from build123d import *

# Parameters (mm, degrees)
SKETCH1_R           = 2.5
SKETCH1_R_2         = 1
BOSS_EXTRUDE1_DEPTH = 4


with BuildPart() as part:
    # Sketch1 → Boss-Extrude1 (new body)
    with BuildSketch(Plane.XY):
        with BuildLine():
            ThreePointArc((15.254156194, 5.023677433), (14.359298867, 11.726874121), (7.604193017, 11.407248683))
            add(Edge.make_bspline(
                [(7.604193017, 11.407248683), (-64.624332124, -68.096129446), (-64.220975839, -174.388465928)],
                knots=[0, 0, 0, 1, 1, 1], degree=2))
            ThreePointArc((-64.220975839, -174.388465928), (-49.220975839, -189.388465928), (-34.220975839, -174.388465928))
            add(Edge.make_bspline(
                [(15.254156194, 5.023677433), (-28.824565765, -79.354910708), (-34.220975839, -174.388465928)],
                knots=[0, 0, 0, 1, 1, 1], degree=2))
        make_face()
        with Locations((11.155830006, 7.88789154)):
            Circle(SKETCH1_R, mode=Mode.SUBTRACT)
        with Locations((-34.220975839, -82.261849143)):
            Circle(SKETCH1_R_2, mode=Mode.SUBTRACT)
        with Locations((-49.220975839, -174.388465928)):
            Circle(SKETCH1_R, mode=Mode.SUBTRACT)
    extrude(amount=BOSS_EXTRUDE1_DEPTH)


solid = part.part
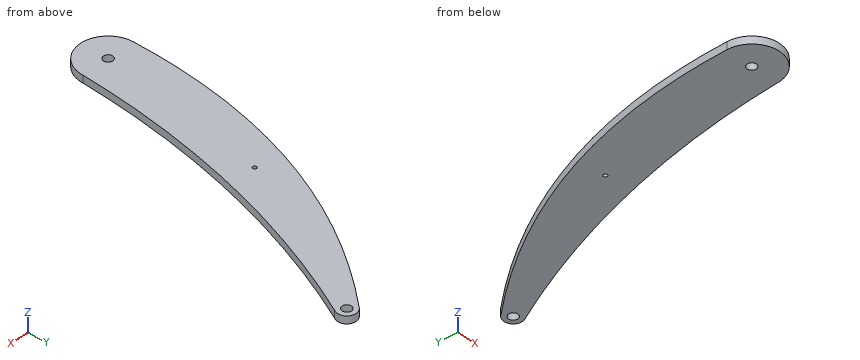
Read the model definition and answer for the solid it produces. Units are mm, in the model's axes. Give positions to 0.01 mm unless a question says otherwise; leave off trailing zeros. Answer in a Markdown table with one row per item. Add a question column.
Item 1: Flat-ended cylindrical pins translate along their axes: P1, Ø5, axis at x = -53, y = -152, coming from the -Z side; P2, Ø1, axis at x = -53.5, z = 1.5, coming from the -Y side; P3, Ø1, axis at y = -109, z = 3, coming from the -X side. Find the tip coordinate at first contact, or state that the pin passes through.
Item 2: Find the intervals of material crossed by L1, parallel to Y at x = 9, z = 3.3; L2, parallel to X at y = -112, z = 0.65; L3, parallel to X at y = -16, z = 3.5, in increasing order.
Item 3: Section A-A, the plane z = 2.3 is taken. Count the separate pieces of the cut face and the enclosed holes in it, and give its area (3 significant figures).
Recorded:
| question | item | result |
|---|---|---|
| 1 | P1 | stops at z = 0 |
| 1 | P2 | stops at y = -188.9 |
| 1 | P3 | stops at x = -57.13 |
| 2 | L1 | y = -7.4 to 6.62, 9.15 to 12.4 |
| 2 | L2 | x = -57.7 to -26.28 |
| 2 | L3 | x = -14.57 to 4.95 |
| 3 | separate pieces | 1 |
| 3 | enclosed holes | 3 |
| 3 | area | 5,300 mm2 |
